Autodesk Inventor part; units mm, degrees
ref_plane "YZ Plane" through (0, 0, 0) normal (1, 0, 0) x (0, 1, 0)
ref_plane "XZ Plane" through (0, 0, 0) normal (0, 1, 0) x (-1, 0, 0)
ref_plane "XY Plane" through (0, 0, 0) normal (0, 0, 1) x (1, 0, 0)
sketch "Sketch1" plane through (0, 0, 0) normal (0, 0, 1) x (1, 0, 0)
  line L0 (0, 0) -> (25.4, 0)
  line L1 (25.4, 0) -> (25.4, 50.8)
  line L2 (25.4, 50.8) -> (0, 50.8)
  line L3 (0, 50.8) -> (0, 0)
  line L4 (1.5875, 1.5875) -> (23.8125, 1.5875)
  line L5 (23.8125, 1.5875) -> (23.8125, 49.2125)
  line L6 (23.8125, 49.2125) -> (1.5875, 49.2125)
  line L7 (1.5875, 49.2125) -> (1.5875, 1.5875)
  dimension "d0" = 25.4
  dimension "d1" = 50.8
  dimension "d2" = 1.5875
  dimension "d3" = 1.5875
  dimension "d4" = 1.5875
  dimension "d5" = 1.5875
extrude "Box Beam Profile" add sketch "Sketch1" along normal blind 101.6
sketch "Sketch2" plane through (25.4, 0, 0) normal (1, 0, 0) x (0, 0, -1)
  line L0 (0, 50.8) -> (-101.6, 50.8)
  line L1 (-101.6, 0) -> (-101.6, 50.8)
  line L2 (0, 0) -> (-101.6, 0)
  line L3 (-101.6, 31.75) -> (-69.85, 0)
  line L4 (-101.6, 31.75) -> (-82.55, 31.75)
  line L5 (-82.55, 31.75) -> (-82.55, 50.8)
  dimension "d8" = 45
  dimension "d9" = 19.05
  dimension "d10" = 19.05
extrude "Through Cutouts" cut sketch "Sketch2" against normal through all
equation "\"d3\" = d2"
equation "\"d4\" = d2"
equation "\"d5\" = d2"
equation "\"d10\" = d9"
properties part number "Bumper Rail Stand" material "Aluminum 6061"
Geometry: final body of the model. Coordinates: model frame, mm. A direction names the side the tool comes from. Give positions to 0.01 mm unless a question says otherwise; leave off trailing zeros. Loops run counter-clockwise (first coordinate to the right, second up) from the corner with the lowest first, then second, coordinate; pieces in that order, holes last. Notation, with made-up numbers: (67.25, 53) - (74.25, 53) arc R30 ccw to (74.25, 92) - close; hole circle Ø2 at (19.5, -40). An arc over 180 degrees is marked (long way). Answer as CSV lines item,"result". Start each with the question number.
1. Pin query (flat end, axial travel): P1, Ø0.8, axis at x = 1, z = 96.5, coming from the +Y side; P2, Ø1, axis at x = 4, y = 31.5, coming from the -Z side; P3, Ø14.5, axis at y = 26.5, z = 42.5, coming from the -X side. Return the tip coordinate at first contact, or that it passes through.
2. Draft query along Y for faces 4 (the face through (23.812, 25, 39)), 5 (the face through (13, 0, 34)), 6 (the face through (1.588, 26, 39)), 7 (the face through (1, 27, 0)). Return one class per face: released by +Y, released by -Y, zero draft, split by the parting line, or undercut.
3. Reachability of faces 1 (the face through (13, 49.212, 41)), 2 (the face through (11, 50, 82.55)), 3 (the face through (25.4, 25, 39)) from +Z, -Z, +X, -X, +Y, -Y: full face, straight path, thin tool, end or side. Return the list, or none.
4. Section C-C, the plane z = 12. Return loops of the section in (x, y), plus the area to 3 significant figures.
5. Section B-B, the plane y = 34.5. Return loops of the section in (x, z), plus the area to 3 significant figures.
6. Section A-A, the plane z = 93. Return loops of the section in (x, y).
7. Section D-D, the plane z = 75.5. Return loops of the section in (x, y).
8. Ray query, L1, parallel to Y at x = 3, z = 36; L2, parallel to X at y = 2, z = 49; L3, parallel to Y at x = 6.75, z = 73.5. Return the intervals inside material, ascending.
Answers:
1,P1,"stops at y = 31.75"
1,P2,"passes through"
1,P3,"stops at x = 0"
2,face 4,"undercut"
2,face 5,"released by -Y"
2,face 6,"undercut"
2,face 7,"zero draft"
3,face 1,"+Z, -Z"
3,face 2,"+Z, +X, -X, +Y"
3,face 3,"+Z, -Z, +X, +Y, -Y"
4,outline,"(0, 0) - (25.4, 0) - (25.4, 50.8) - (0, 50.8) - close; hole (1.59, 1.59) - (23.81, 1.59) - (23.81, 49.21) - (1.59, 49.21) - close"
4,area,"232 mm2"
5,outline,"(0, 0) - (1.59, 0) - (1.59, 82.55) - (0, 82.55) - close; (23.81, 0) - (25.4, 0) - (25.4, 82.55) - (23.81, 82.55) - close"
5,area,"262 mm2"
6,outline,"(0, 23.15) - (1.59, 23.15) - (1.59, 31.75) - (0, 31.75) - close; (23.81, 23.15) - (25.4, 23.15) - (25.4, 31.75) - (23.81, 31.75) - close"
7,outline,"(0, 5.65) - (1.59, 5.65) - (1.59, 49.21) - (23.81, 49.21) - (23.81, 5.65) - (25.4, 5.65) - (25.4, 50.8) - (0, 50.8) - close"
8,L1,"y = 0 to 1.59, 49.21 to 50.8"
8,L2,"x = 0 to 1.59, 23.81 to 25.4"
8,L3,"y = 49.21 to 50.8"
